Autodesk Fusion 360 part; units mm, degrees
sketch "Sketch1" plane through (0, 0, 0) normal (0, 0, 1) x (1, 0, 0)
  line L0 (68.541, -12.5) -> (-110, -12.5) construction
  line L1 (-20.75, -50) -> (-20.75, 25) construction
  point P0 (-20.75, -12.5)
sketch "Sketch2" plane through (0, 0, 0) normal (0, 0, 1) x (1, 0, 0)
  line L0 (54.25, 7.5) -> (-95.75, 7.5)
  line L1 (-95.75, 7.5) -> (-95.75, -32.5)
  line L2 (-95.75, -32.5) -> (54.25, -32.5)
  line L3 (54.25, -32.5) -> (54.25, 7.5)
  line L4 (54.25, 7.5) -> (-95.75, -32.5) construction
  line L5 (-95.75, 7.5) -> (54.25, -32.5) construction
  line L6 (26.6666, -12.5) -> (38.5, -12.5) construction
  circle A0 centre (32.5833, -12.5) radius 2.75
  line L7 (14, -12.5) -> (2.2, -12.5) construction
  circle A1 centre (8.1, -12.5) radius 2.75
  line L8 (-49.1, -12.5) -> (-52.4, -12.5) construction
  circle A2 centre (-52.4, -12.5) radius 2.75
  line L9 (-73.1, -12.5) -> (-69.8, -12.5) construction
  circle A3 centre (-69.8, -12.5) radius 2.75
  point P0 (-20.75, -12.5)
  dimension "d1" = 150
  dimension "d2" = 40
  dimension "d3" = 5.5
  dimension "d4" = 5.5
  dimension "d5" = 3.3
  dimension "d6" = 5.5
  dimension "d7" = 3.3
  dimension "d8" = 5.5
extrude "Extrude1" add sketch "Sketch2" along normal blind 2.5
sketch "Sketch3" plane through (0, 0, 2.5) normal (0, 0, 1) x (-1, 0, 0)
  circle A0 centre (-32.5833, 12.5) radius 2.75
  circle A1 centre (69.8, 12.5) radius 2.75
  circle A2 centre (-8.1, 12.5) radius 2.75
  circle A3 centre (52.4, 12.5) radius 2.75
  line L0 (-54.25, 32.5) -> (-54.25, -7.5)
  line L1 (-54.25, -7.5) -> (95.75, -7.5)
  line L2 (95.75, -7.5) -> (95.75, 32.5)
  line L3 (95.75, 32.5) -> (-54.25, 32.5)
sketch "Sketch4" plane through (0, 0, 2.5) normal (0, 0, 1) x (-1, 0, 0)
  line L0 (-29.8338, 12.5) -> (-35.3337, 12.5) construction
  line L1 (-39.2087, 4.875) -> (-25.9587, 4.875)
  line L2 (-25.9587, 4.875) -> (-25.9587, 20.125)
  line L3 (-25.9587, 20.125) -> (-39.2087, 20.125)
  line L4 (-39.2087, 20.125) -> (-39.2087, 4.875)
  line L5 (-39.2087, 4.875) -> (-25.9587, 20.125) construction
  line L6 (-25.9587, 4.875) -> (-39.2087, 20.125) construction
  line L7 (-41.2087, 2.875) -> (-23.9587, 2.875)
  line L8 (-23.9587, 2.875) -> (-23.9587, 22.125)
  line L9 (-23.9587, 22.125) -> (-41.2087, 22.125)
  line L10 (-41.2087, 22.125) -> (-41.2087, 2.875)
  line L11 (-41.2087, 2.875) -> (-23.9587, 22.125) construction
  line L12 (-23.9587, 2.875) -> (-41.2087, 22.125) construction
  line L13 (-39.2087, 12.5) -> (-39.2087, 9)
  line L14 (-39.2087, 9) -> (-41.2087, 9)
  line L15 (-41.2087, 9) -> (-41.2087, 16)
  line L16 (-41.2087, 16) -> (-39.2087, 16)
  line L17 (-39.2087, 16) -> (-39.2087, 12.5)
  line L18 (-5.35, 12.5) -> (-10.85, 12.5) construction
  line L19 (-14.725, 4.875) -> (-1.475, 4.875)
  line L20 (-1.475, 4.875) -> (-1.475, 20.125)
  line L21 (-1.475, 20.125) -> (-14.725, 20.125)
  line L22 (-14.725, 20.125) -> (-14.725, 4.875)
  line L23 (-14.725, 4.875) -> (-1.475, 20.125) construction
  line L24 (-1.475, 4.875) -> (-14.725, 20.125) construction
  line L25 (-16.725, 2.875) -> (0.525, 2.875)
  line L26 (0.525, 2.875) -> (0.525, 22.125)
  line L27 (0.525, 22.125) -> (-16.725, 22.125)
  line L28 (-16.725, 22.125) -> (-16.725, 2.875)
  line L29 (-16.725, 2.875) -> (0.525, 22.125) construction
  line L30 (0.525, 2.875) -> (-16.725, 22.125) construction
  line L31 (-1.475, 16) -> (-1.475, 9)
  line L32 (0.525, 16) -> (0.525, 9)
  line L33 (0.525, 9) -> (-1.475, 9)
  line L34 (0.525, 16) -> (-1.475, 16)
  line L35 (55.15, 12.5) -> (49.65, 12.5) construction
  line L36 (45.775, 4.875) -> (59.025, 4.875)
  line L37 (59.025, 4.875) -> (59.025, 20.125)
  line L38 (59.025, 20.125) -> (45.775, 20.125)
  line L39 (45.775, 20.125) -> (45.775, 4.875)
  line L40 (45.775, 4.875) -> (59.025, 20.125) construction
  line L41 (59.025, 4.875) -> (45.775, 20.125) construction
  line L42 (61.025, 22.125) -> (43.775, 22.125)
  line L43 (43.775, 22.125) -> (43.775, 2.875)
  line L44 (43.775, 2.875) -> (61.025, 2.875)
  line L45 (61.025, 22.125) -> (43.775, 2.875) construction
  line L46 (43.775, 22.125) -> (61.025, 2.875) construction
  line L47 (72.55, 12.5) -> (67.05, 12.5) construction
  line L48 (63.175, 4.875) -> (76.425, 4.875)
  line L49 (76.425, 4.875) -> (76.425, 20.125)
  line L50 (76.425, 20.125) -> (63.175, 20.125)
  line L51 (63.175, 20.125) -> (63.175, 4.875)
  line L52 (63.175, 4.875) -> (76.425, 20.125) construction
  line L53 (76.425, 4.875) -> (63.175, 20.125) construction
  line L54 (61.175, 2.875) -> (78.425, 2.875)
  line L55 (78.425, 2.875) -> (78.425, 22.125)
  line L56 (78.425, 22.125) -> (61.175, 22.125)
  line L57 (61.175, 2.875) -> (78.425, 22.125) construction
  line L58 (78.425, 2.875) -> (61.175, 22.125) construction
  line L59 (61.175, 2.875) -> (61.025, 2.875)
  line L60 (61.175, 22.125) -> (61.025, 22.125)
  line L61 (43.775, 16) -> (43.775, 9)
  line L62 (45.775, 16) -> (45.775, 9)
  line L63 (45.775, 9) -> (43.775, 9)
  line L64 (45.775, 16) -> (43.775, 16)
  line L65 (76.425, 16) -> (76.425, 9)
  line L66 (78.425, 16) -> (78.425, 9)
  line L67 (78.425, 9) -> (76.425, 9)
  line L68 (76.425, 16) -> (78.425, 16)
  point P0 (-32.5837, 12.5)
  point P1 (-32.5837, 12.5)
  point P2 (-8.1, 12.5)
  point P3 (-8.1, 12.5)
  point P4 (-1.475, 12.5)
  point P5 (0.525, 12.5)
  point P6 (52.4, 12.5)
  point P7 (52.4, 12.5)
  point P8 (69.8, 12.5)
  point P9 (69.8, 12.5)
  point P10 (43.775, 12.5)
  point P11 (45.775, 12.5)
  point P12 (76.425, 12.5)
  point P13 (78.425, 12.5)
  dimension "d11" = 13.25
  dimension "d12" = 15.25
  dimension "d13" = 17.25
  dimension "d14" = 19.25
  dimension "d15" = 3.5
  dimension "d16" = 7
  dimension "d17" = 13.25
  dimension "d18" = 15.25
  dimension "d19" = 17.25
  dimension "d20" = 19.25
  dimension "d21" = 7
  dimension "d22" = 7
  dimension "d23" = 13.25
  dimension "d24" = 15.25
  dimension "d25" = 17.25
  dimension "d26" = 19.25
  dimension "d27" = 13.25
  dimension "d28" = 15.25
  dimension "d29" = 17.25
  dimension "d30" = 19.25
  dimension "d31" = 7
  dimension "d32" = 7
  dimension "d33" = 7
  dimension "d34" = 7
extrude "Extrude2" add sketch "Sketch4" along normal blind 12 contours L1 L2 L3 L4 L7 L8 L9 L10 L14 L16 | L19 L20 L21 L22 L25 L26 L27 L28 L33 L34 | L36 L37 L38 L39 L42 L43 L44 L48 L49 L50 L51 L54 L55 L56 L59 L60 L63 L64 L67 L68
sketch "Sketch5" plane through (0, 0, 2.5) normal (0, 0, 1) x (-1, 0, 0)
sketch "Sketch7" plane through (54.25, 0, 0) normal (1, 0, 0) x (0, 1, 0)
  line L0 (-32.5, 0) -> (7.5, 0)
  line L1 (7.5, 0) -> (7.5, 2.5)
  line L2 (7.5, 2.5) -> (-32.5, 2.5)
  line L3 (-32.5, 2.5) -> (-32.5, 0)
  line L4 (-25, 2.5) -> (0, 2.5)
  line L5 (-21.5, 2.5) -> (-3.5, 2.5)
  line L6 (-12.5, 7.5) -> (-3.5, 7.5)
  line L7 (-3.5, 7.5) -> (0, 2.5)
  line L8 (-12.5, 7.5) -> (-21.5, 7.5)
  line L9 (-21.5, 7.5) -> (-25, 2.5)
  line L10 (-12.5, 2.5) -> (-12.5, 7.5) construction
  circle A0 centre (-12.5, 5) radius 1.1
  point P0 (-12.5, 2.5)
  point P1 (-12.5, 2.5)
  dimension "d39" = 25
  dimension "d40" = 18
  dimension "d41" = 2.2
extrude "Extrude3" add sketch "Sketch7" against normal blind 2.5 contours L2 L4 L5 L6 L7 L8 L9
sketch "Sketch8" plane through (-95.75, 0, 0) normal (-1, 0, 0) x (0, -1, 0)
  line L0 (-7.5, 0) -> (32.5, 0)
  line L1 (32.5, 0) -> (32.5, 2.5)
  line L2 (32.5, 2.5) -> (-7.5, 2.5)
  line L3 (-7.5, 2.5) -> (-7.5, 0)
  line L4 (0, 2.5) -> (25, 2.5)
  line L5 (3.5, 7.5) -> (21.5, 7.5)
  line L6 (3.5, 7.5) -> (0, 2.5)
  line L7 (21.5, 7.5) -> (25, 2.5)
  circle A0 centre (12.5, 5) radius 1.1
  point P0 (12.5, 2.5)
  dimension "d44" = 25
  dimension "d46" = 18
  dimension "d47" = 2.2
extrude "Extrude4" add sketch "Sketch8" against normal blind 2.5 contours L2 L4 L5 L6 L7
fillet "Fillet1" radius 1 4 edges at (-94.5, -21.5, 7.5) (-94.5, -25, 2.5) (-94.5, -3.5, 7.5) (-94.5, 0, 2.5)
fillet "Fillet2" radius 1 4 edges at (53, -25, 2.5) (53, -21.5, 7.5) (53, -3.5, 7.5) (53, 0, 2.5)
fillet "Fillet3" radius 0.5 5 edges at (41.2087, -19.0625, 2.5) (32.5837, -22.125, 2.5) (41.2087, -5.9375, 2.5) (32.5837, -2.875, 2.5) (23.9587, -12.5, 2.5)
fillet "Fillet4" radius 0.5 15 edges at (16.725, -12.5, 2.5) (8.1, -2.875, 2.5) (8.1, -22.125, 2.5) (-0.525, -5.9375, 2.5) (-0.525, -19.0625, 2.5) (-52.4, -22.125, 2.5) (-61.1, -22.125, 2.5) (-69.8, -22.125, 2.5) (-78.425, -19.0625, 2.5) (-78.425, -5.9375, 2.5) (-43.775, -19.0625, 2.5) (-43.775, -5.9375, 2.5) (-69.8, -2.875, 2.5) (-61.1, -2.875, 2.5) (-52.4, -2.875, 2.5)
fillet "Fillet5" radius 1 8 edges at (-45.775, -16, 8.5) (-45.775, -9, 8.5) (-76.425, -9, 8.5) (-76.425, -16, 8.5) (1.475, -16, 8.5) (1.475, -9, 8.5) (39.2087, -16, 8.5) (39.2087, -9, 8.5)
Check sheet for the modelled part. Datum: model origin and axes. Units: mm. A direction names the side the tool comes from. Round coordinates to 2 decimals unless told otherwise and drop trailing zeros. Order: outer loops, then holes, each group sorted by start corner. A loop starts at its lowest first (then second) coordinate and runs counter-clockwise, first axis right, second up.
(1) Cross-section at C-C, the plane x = 28. Enter the section's corners in (y, z) (3 decimals), and give its area (3 significant figures).
(2) Go/stop test with flat-tipped pins: P1, Ø3, axis at x = -94, y = -16, coming from the +Z side; P2, Ø1.6, axis at x = -78.5, z = 8.5, coming from the -Y side (3 decimals); P3, Ø0.8, axis at x = -0.5, z = 8.5, coming from the +Y side (3 decimals); P4, Ø6, axis at y = 1.5, z = 7, coming from the -X side. Record where each tip stops, or that it passes through.
(3) Scan lines: probe 1 along X at (y, z) = (-4, 8.5) (3 decimals); probe 2 along X at (y, z) = (-23.5, 4.5); probe 3 along Y at (x, z) = (29, 5) (3 decimals). Record each from-to range of solid material in increasing order.
(4) Cross-section at A-A, the plane x = -69.8. Enter the section's corners in (y, z) (3 decimals).
(5) Draft check along X on faces 5 (the flat face through (-78.425, -19, 9)), 6 (the flat face through (-22, -32.5, 1)), 7 (the flat face through (-76.425, -6, 8)). Enter one of: pulls with the +X half, pulls with the -X half, needs draft (parallel to the pull), parting line crosses it, or undercut.
(6) Cross-section at B-B, the plane z = 9.5. State how many separate pieces and enclosed holes the cut face has, and give its area (3 significant figures).
(7) Access from +Z, -Z, +X, -X, +Y, -Y to the whole of each face (thin tool, end or side, straight path). Record for faces 1 (the flat face through (-76.425, -19, 8)), 2 (the flat face through (-95, -12, 7.5)), 3 (the flat face through (-43.775, -19, 9)), 4 (the cylindrical face through (10.72, -13.33, 1.23)).
(8) Cross-section at D-D, the plane y = 2. Enter the section's corners in (x, z), and give its area (3 significant figures).
Check sheet entries:
1. outline: (-32.5, 0) - (7.5, 0) - (7.5, 2.5) - (-2.375, 2.5) arc R0.5 cw to (-2.875, 3) - (-2.875, 14.5) - (-4.875, 14.5) - (-4.875, 2.5) - (-20.125, 2.5) - (-20.125, 14.5) - (-22.125, 14.5) - (-22.125, 3) arc R0.5 cw to (-22.625, 2.5) - (-32.5, 2.5) - close
1. area: 148 mm2
2. P1: stops at z = 7.5
2. P2: stops at y = -22.125
2. P3: stops at y = -2.875
2. P4: passes through
3. probe 1: x = -78.425 to -43.775, -0.525 to 16.725, 23.959 to 41.209
3. probe 2: x = -95.75 to -93.25, 51.75 to 54.25
3. probe 3: y = -22.125 to -20.125, -4.875 to -2.875
4. outline: (-32.5, 0) - (-15.25, 0) - (-15.25, 2.5) - (-20.125, 2.5) - (-20.125, 14.5) - (-22.125, 14.5) - (-22.125, 3) arc R0.5 cw to (-22.625, 2.5) - (-32.5, 2.5) - close; (-9.75, 0) - (7.5, 0) - (7.5, 2.5) - (-2.375, 2.5) arc R0.5 cw to (-2.875, 3) - (-2.875, 14.5) - (-4.875, 14.5) - (-4.875, 2.5) - (-9.75, 2.5) - close
5. face 5: undercut
5. face 6: needs draft
5. face 7: undercut
6. separate pieces: 3
6. enclosed holes: 0
6. area: 465 mm2
7. face 1: +Z
7. face 2: +Z, -X, +Y, -Y
7. face 3: +Z, +Y, -Y
7. face 4: +Z, -Z
8. outline: (-95.75, 0) - (54.25, 0) - (54.25, 2.5) - (-95.75, 2.5) - close
8. area: 375 mm2
